from build123d import *

# Parameters (mm, degrees)
MAIN_WEB_PROFILE_W                             = 60
MAIN_WEB_PROFILE_H                             = 14
MAIN_WEB_DEPTH                                 = 4
SHOULDER_HORN_FLANGE_PROFILE_R                 = 16
SHOULDER_HORN_FLANGE_DEPTH                     = 4
ELBOW_SERVO_MOUNT_PROFILE_W                    = 48
ELBOW_SERVO_MOUNT_PROFILE_H                    = 28
ELBOW_SERVO_MOUNT_DEPTH                        = 4
SG90_BODY_CLEARANCE_START                      = -5
SG90_BODY_CLEARANCE_PROFILE_W                  = 23.8
SG90_BODY_CLEARANCE_PROFILE_H                  = 13
SG90_BODY_CLEARANCE_DEPTH                      = 97.49863387
ELBOW_TAB_FASTENERS_START                      = -50
ELBOW_TAB_FASTENERS_PROFILE_R                  = 1.3
ELBOW_TAB_FASTENERS_DEPTH                      = 142.49863387
SHOULDER_CENTER_SCREW_ACCESS_START             = -50
SHOULDER_CENTER_SCREW_ACCESS_PROFILE_R         = 4
SHOULDER_CENTER_SCREW_ACCESS_DEPTH             = 142.49863387
CABLE_TIE_HOLES_START                          = -50
CABLE_TIE_HOLES_PROFILE_R                      = 1.6
CABLE_TIE_HOLES_DEPTH                          = 142.49863387
PASSIVE_LOWER_MOUNT_BOSS_PROFILE_R             = 5
PASSIVE_LOWER_MOUNT_BOSS_DEPTH                 = 4
PASSIVE_UPPER_MOUNT_BOSS_PROFILE_R             = 5
PASSIVE_UPPER_MOUNT_BOSS_DEPTH                 = 4
PASSIVE_CHEEK_STANDOFFS_START                  = -50
PASSIVE_CHEEK_STANDOFFS_PROFILE_R              = 1.6
PASSIVE_CHEEK_STANDOFFS_DEPTH                  = 142.49863387
SHOULDER_DOWEL_SUPPORT_HUB_START               = 4
SHOULDER_DOWEL_SUPPORT_HUB_PROFILE_R           = 7
SHOULDER_DOWEL_SUPPORT_HUB_PROFILE_R_2         = 4
SHOULDER_DOWEL_SUPPORT_HUB_DEPTH               = 4
RAISED_M3_WASHER_SEATS_HEIGHT8_START           = 4
RAISED_M3_WASHER_SEATS_PCD14_PROFILE_R         = 3.5
RAISED_M3_WASHER_SEATS_HEIGHT8_DEPTH           = 4
METAL_HORN_M3_CLEARANCE_PCD14_START            = -50
METAL_HORN_M3_CLEARANCE_PCD14_PROFILE_R        = 1.6
METAL_HORN_M3_CLEARANCE_PCD14_DEPTH            = 142.760557976
RESTORE_SHOULDER_SLEEVE_BORE_START             = -50
RESTORE_SHOULDER_SLEEVE_BORE_PROFILE_R         = 4
RESTORE_SHOULDER_SLEEVE_BORE_DEPTH             = 142.760557976
FILLET1_R                                      = 7.5
LARGER_ELBOW_SERVO_MOUNT_REPLACES_SG_2_W       = 58
LARGER_ELBOW_SERVO_MOUNT_REPLACES_SG_2_H       = 30
LARGER_ELBOW_SERVO_MOUNT_REPLACES_SG90_O_DEPTH = 4
MG996R_ELBOW_BODY_CLEARANCE_START              = -5
MG996R_ELBOW_BODY_CLEARANCE_PROFILE_W          = 41.7
MG996R_ELBOW_BODY_CLEARANCE_PROFILE_H          = 20.7
MG996R_ELBOW_BODY_CLEARANCE_DEPTH              = 107.587400794
MG996R_ELBOW_TAB_FASTENERS_START               = -50
MG996R_ELBOW_TAB_FASTENERS_PROFILE_R           = 1.5
MG996R_ELBOW_TAB_FASTENERS_DEPTH               = 152.587400794
FILLET2_R                                      = 10


with BuildPart() as part:
    # Main_web_profile → Main_web (new body)
    with BuildSketch(Plane.XY):
        with Locations((30, 0)):
            Rectangle(MAIN_WEB_PROFILE_W, MAIN_WEB_PROFILE_H)
    extrude(amount=MAIN_WEB_DEPTH)

    # Shoulder_horn_flange_profile → Shoulder_horn_flange (add)
    with BuildSketch(Plane.XY):
        Circle(SHOULDER_HORN_FLANGE_PROFILE_R)
    extrude(amount=SHOULDER_HORN_FLANGE_DEPTH)

    # Elbow_servo_mount_profile → Elbow_servo_mount (add)
    with BuildSketch(Plane.XY):
        with Locations((66, 0)):
            Rectangle(ELBOW_SERVO_MOUNT_PROFILE_W, ELBOW_SERVO_MOUNT_PROFILE_H)
    extrude(amount=ELBOW_SERVO_MOUNT_DEPTH)

    # SG90_body_clearance_profile → SG90_body_clearance (cut, through all)
    with BuildSketch(Plane.XY.offset(SG90_BODY_CLEARANCE_START)):
        with Locations((65.5, 0)):
            Rectangle(SG90_BODY_CLEARANCE_PROFILE_W, SG90_BODY_CLEARANCE_PROFILE_H)
    extrude(amount=SG90_BODY_CLEARANCE_DEPTH, mode=Mode.SUBTRACT)

    # Elbow_tab_fasteners_profile → Elbow_tab_fasteners (cut, through all)
    with BuildSketch(Plane.XY.offset(ELBOW_TAB_FASTENERS_START)):
        with Locations(Location((51, 0, 0), (0, 0, 180))):
            Circle(ELBOW_TAB_FASTENERS_PROFILE_R)
        with Locations(Location((80, 0, 0), (0, 0, 180))):
            Circle(ELBOW_TAB_FASTENERS_PROFILE_R)
    extrude(amount=ELBOW_TAB_FASTENERS_DEPTH, mode=Mode.SUBTRACT)

    # Shoulder_center_screw_access_profile → Shoulder_center_screw_access (cut, through all)
    with BuildSketch(Plane.XY.offset(SHOULDER_CENTER_SCREW_ACCESS_START)):
        with Locations(Location((0, 0, 0), (0, 0, 180))):
            Circle(SHOULDER_CENTER_SCREW_ACCESS_PROFILE_R)
    extrude(amount=SHOULDER_CENTER_SCREW_ACCESS_DEPTH, mode=Mode.SUBTRACT)

    # Cable_tie_holes_profile → Cable_tie_holes (cut, through all)
    with BuildSketch(Plane.XY.offset(CABLE_TIE_HOLES_START)):
        with Locations(Location((27, -3, 0), (0, 0, 180))):
            Circle(CABLE_TIE_HOLES_PROFILE_R)
        with Locations(Location((27, 3, 0), (0, 0, 180))):
            Circle(CABLE_TIE_HOLES_PROFILE_R)
    extrude(amount=CABLE_TIE_HOLES_DEPTH, mode=Mode.SUBTRACT)

    # Passive_lower_mount_boss_profile → Passive_lower_mount_boss (add)
    with BuildSketch(Plane.XY):
        with Locations((35, -9)):
            Circle(PASSIVE_LOWER_MOUNT_BOSS_PROFILE_R)
    extrude(amount=PASSIVE_LOWER_MOUNT_BOSS_DEPTH)

    # Passive_upper_mount_boss_profile → Passive_upper_mount_boss (add)
    with BuildSketch(Plane.XY):
        with Locations((35, 9)):
            Circle(PASSIVE_UPPER_MOUNT_BOSS_PROFILE_R)
    extrude(amount=PASSIVE_UPPER_MOUNT_BOSS_DEPTH)

    # Passive_cheek_standoffs_profile → Passive_cheek_standoffs (cut, through all)
    with BuildSketch(Plane.XY.offset(PASSIVE_CHEEK_STANDOFFS_START)):
        with Locations(Location((35, -9, 0), (0, 0, 180))):
            Circle(PASSIVE_CHEEK_STANDOFFS_PROFILE_R)
        with Locations(Location((35, 9, 0), (0, 0, 180))):
            Circle(PASSIVE_CHEEK_STANDOFFS_PROFILE_R)
    extrude(amount=PASSIVE_CHEEK_STANDOFFS_DEPTH, mode=Mode.SUBTRACT)

    # Shoulder_dowel_support_hub_profile → Shoulder_dowel_support_hub (add)
    with BuildSketch(Plane.XY.offset(SHOULDER_DOWEL_SUPPORT_HUB_START)):
        Circle(SHOULDER_DOWEL_SUPPORT_HUB_PROFILE_R)
        with Locations(Location((0, 0, 0), (0, 0, 180))):
            Circle(SHOULDER_DOWEL_SUPPORT_HUB_PROFILE_R_2, mode=Mode.SUBTRACT)
    extrude(amount=SHOULDER_DOWEL_SUPPORT_HUB_DEPTH)

    # Raised_M3_washer_seats_PCD14_profile → Raised_M3_washer_seats_height8 (add)
    with BuildSketch(Plane.XY.offset(RAISED_M3_WASHER_SEATS_HEIGHT8_START)):
        with Locations((7, 0)):
            Circle(RAISED_M3_WASHER_SEATS_PCD14_PROFILE_R)
        with Locations((-7, 0)):
            Circle(RAISED_M3_WASHER_SEATS_PCD14_PROFILE_R)
        with Locations((0, 7)):
            Circle(RAISED_M3_WASHER_SEATS_PCD14_PROFILE_R)
        with Locations((0, -7)):
            Circle(RAISED_M3_WASHER_SEATS_PCD14_PROFILE_R)
    extrude(amount=RAISED_M3_WASHER_SEATS_HEIGHT8_DEPTH)

    # Metal_horn_M3_clearance_PCD14_profile → Metal_horn_M3_clearance_PCD14 (cut, through all)
    with BuildSketch(Plane.XY.offset(METAL_HORN_M3_CLEARANCE_PCD14_START)):
        with Locations(Location((7, 0, 0), (0, 0, 180))):
            Circle(METAL_HORN_M3_CLEARANCE_PCD14_PROFILE_R)
        with Locations(Location((-7, 0, 0), (0, 0, 180))):
            Circle(METAL_HORN_M3_CLEARANCE_PCD14_PROFILE_R)
        with Locations(Location((0, 7, 0), (0, 0, 180))):
            Circle(METAL_HORN_M3_CLEARANCE_PCD14_PROFILE_R)
        with Locations(Location((0, -7, 0), (0, 0, 180))):
            Circle(METAL_HORN_M3_CLEARANCE_PCD14_PROFILE_R)
    extrude(amount=METAL_HORN_M3_CLEARANCE_PCD14_DEPTH, mode=Mode.SUBTRACT)

    # Restore_shoulder_sleeve_bore_profile → Restore_shoulder_sleeve_bore (cut, through all)
    with BuildSketch(Plane.XY.offset(RESTORE_SHOULDER_SLEEVE_BORE_START)):
        with Locations(Location((0, 0, 0), (0, 0, 180))):
            Circle(RESTORE_SHOULDER_SLEEVE_BORE_PROFILE_R)
    extrude(amount=RESTORE_SHOULDER_SLEEVE_BORE_DEPTH, mode=Mode.SUBTRACT)

    # Fillet1
    # the kernel refuses this fillet: 7.5 mm, written as the material it takes off along each edge
    with BuildSketch(Plane(origin=(42, -14, -18.708286934), x_dir=(0, 1, 0), z_dir=(0, 0, 1))) as fillet1_piece_1:
        with BuildLine():
            CenterArc((7.5, -7.483314774), FILLET1_R, 93.822553729, 86.177446271)
            Line((0, -7.483314774), (-0.15, -7.483314774))
            Line((-0.15, -7.483314774), (-0.15, 0))
            Line((-0.15, 0), (0, 0.15))
            ThreePointArc((0, 0.15), (3.5, 0.15), (6.99, 0.149666295))
            Line((6.99, 0.149666295), (7, 0))
        make_face()
    extrude(amount=41.416573868, mode=Mode.SUBTRACT)
    with BuildSketch(Plane(origin=(90, -14, -18.75), x_dir=(-1, 0, 0), z_dir=(0, 0, 1)), Plane(origin=(90, 14, -18.75), x_dir=(0, -1, 0), z_dir=(0, 0, 1))) as fillet1_piece_2:
        with BuildLine():
            CenterArc((FILLET1_R, -FILLET1_R), FILLET1_R, 90, 90)
            Line((0, -FILLET1_R), (-FILLET1_R * 0.02, -FILLET1_R))
            Line((-FILLET1_R * 0.02, -FILLET1_R), (-FILLET1_R * 0.02, FILLET1_R * 0.02))
            Line((-FILLET1_R * 0.02, FILLET1_R * 0.02), (FILLET1_R, FILLET1_R * 0.02))
            Line((FILLET1_R, FILLET1_R * 0.02), (FILLET1_R, 0))
        make_face()
    extrude(amount=41.5, mode=Mode.SUBTRACT)
    with BuildSketch(Plane(origin=(42, 14, -18.708286934), x_dir=(0, -1, 0), z_dir=(0, 0, 1))) as fillet1_piece_3:
        with BuildLine():
            CenterArc((7.5, 7.483314774), FILLET1_R, 180, 86.177446271)
            Line((0, 7.483314774), (-0.15, 7.483314774))
            Line((-0.15, 7.483314774), (-0.15, 0))
            Line((-0.15, 0), (0, -0.15))
            ThreePointArc((0, -0.15), (3.5, -0.15), (6.99, -0.149666295))
            Line((6.99, -0.149666295), (7, 0))
        make_face()
    extrude(amount=41.416573868, mode=Mode.SUBTRACT)

    # Larger_elbow_servo_mount_replaces_SG 2 → Larger_elbow_servo_mount_replaces_SG90_o (add)
    with BuildSketch(Plane.XY):
        with Locations((71, 0)):
            Rectangle(LARGER_ELBOW_SERVO_MOUNT_REPLACES_SG_2_W, LARGER_ELBOW_SERVO_MOUNT_REPLACES_SG_2_H)
    extrude(amount=LARGER_ELBOW_SERVO_MOUNT_REPLACES_SG90_O_DEPTH)

    # MG996R_elbow_body_clearance_profile → MG996R_elbow_body_clearance (cut, through all)
    with BuildSketch(Plane.XY.offset(MG996R_ELBOW_BODY_CLEARANCE_START)):
        with Locations((70.35, 0)):
            Rectangle(MG996R_ELBOW_BODY_CLEARANCE_PROFILE_W, MG996R_ELBOW_BODY_CLEARANCE_PROFILE_H)
    extrude(amount=MG996R_ELBOW_BODY_CLEARANCE_DEPTH, mode=Mode.SUBTRACT)

    # MG996R_elbow_tab_fasteners_profile → MG996R_elbow_tab_fasteners (cut, through all)
    with BuildSketch(Plane.XY.offset(MG996R_ELBOW_TAB_FASTENERS_START)):
        with Locations(Location((47, -5, 0), (0, 0, 180))):
            Circle(MG996R_ELBOW_TAB_FASTENERS_PROFILE_R)
        with Locations(Location((47, 5, 0), (0, 0, 180))):
            Circle(MG996R_ELBOW_TAB_FASTENERS_PROFILE_R)
        with Locations(Location((94, -5, 0), (0, 0, 180))):
            Circle(MG996R_ELBOW_TAB_FASTENERS_PROFILE_R)
        with Locations(Location((94, 5, 0), (0, 0, 180))):
            Circle(MG996R_ELBOW_TAB_FASTENERS_PROFILE_R)
    extrude(amount=MG996R_ELBOW_TAB_FASTENERS_DEPTH, mode=Mode.SUBTRACT)

    # Fillet2
    # the kernel refuses this fillet: 10 mm, written as the material it takes off along each edge
    with BuildSketch(Plane(origin=(42, 15, -24.494897428), x_dir=(1, 0, 0), z_dir=(0, 0, 1))) as fillet2_piece_1:
        with BuildLine():
            CenterArc((9.797958971, -10), FILLET2_R, 90, 78.463040967)
            Line((0, -8), (-0.195959179, -7.96))
            ThreePointArc((-0.195959179, -7.96), (-0.2, -4), (-0.2, 0))
            Line((-0.2, 0), (0, 0.2))
            Line((0, 0.2), (9.797958971, 0.2))
            Line((9.797958971, 0.2), (9.797958971, 0))
        make_face()
    extrude(amount=52.989794856, mode=Mode.SUBTRACT)
    with BuildSketch(Plane(origin=(42, -15, -24.494897428), x_dir=(0, 1, 0), z_dir=(0, 0, 1))) as fillet2_piece_2:
        with BuildLine():
            CenterArc((10, -9.797958971), FILLET2_R, 101.536959033, 78.463040967)
            Line((0, -9.797958971), (-0.2, -9.797958971))
            Line((-0.2, -9.797958971), (-0.2, 0))
            Line((-0.2, 0), (0, 0.2))
            ThreePointArc((0, 0.2), (4, 0.2), (7.96, 0.195959179))
            Line((7.96, 0.195959179), (8, 0))
        make_face()
    extrude(amount=52.989794856, mode=Mode.SUBTRACT)
    with BuildSketch(Plane(origin=(100, -15, -25), x_dir=(-1, 0, 0), z_dir=(0, 0, 1)), Plane(origin=(100, 15, -25), x_dir=(0, -1, 0), z_dir=(0, 0, 1))) as fillet2_piece_3:
        with BuildLine():
            CenterArc((FILLET2_R, -FILLET2_R), FILLET2_R, 90, 90)
            Line((0, -FILLET2_R), (-FILLET2_R * 0.02, -FILLET2_R))
            Line((-FILLET2_R * 0.02, -FILLET2_R), (-FILLET2_R * 0.02, FILLET2_R * 0.02))
            Line((-FILLET2_R * 0.02, FILLET2_R * 0.02), (FILLET2_R, FILLET2_R * 0.02))
            Line((FILLET2_R, FILLET2_R * 0.02), (FILLET2_R, 0))
        make_face()
    extrude(amount=54, mode=Mode.SUBTRACT)


solid = part.part
For this review, take the finished solid that the model builds, in its own axes (mm). A direction names the side the tool comes from. Round coordinates to 2 decimals unless told otherwise and drop trailing zeros. Write each loop counter-clockwise with the first axis right and the second up, starting at its lowest first coordinate (ties: lowest second). Pieces come first, ordered by that corner, then holes. Notation, with made-up numbers: (-21, 44) -> (8, 44) arc R20 cw to (8, 73) -> close; hole circle Ø8 at (42.5, 37). An arc over 180 degrees is marked (long way). Use CSV: the item, a comma, the result in double quotes.
(1) For faces 5 (the face through (97.15, 11.99, 1.97)), 6 (the face through (10.5, -0.1, 6)), 7 (the face through (70, -10.35, 2)), list the 3-axis set-ups (+Z, -Z, +X, -X, +Y, -Y) from which the entire face can be reached by the end or side of a thin tool; tool diameter is ignored.
Computed values:
face 5,"+Z, -Z, +X, +Y"
face 6,"+Z"
face 7,"+Z, -Z"
(2) Clearance check with flat-ended pins moving along their axes: P1, Ø1.5, axis at x = 68.5, z = 1, coming from the -Y side; P2, Ø16, axis at x = 38, y = -0.5, coming from the +Z side; P3, Ø1.2, axis at x = 75.5, z = 1.5, coming from the +Y side. State where each tip first meets the part, or that it passes through.
Computed values:
P1,"y = -15"
P2,"z = 4"
P3,"y = 15"
(3) To check wall thickness, follow L1, parallel to Y at x = 79.5, z = 3; L2, parallel to Y at x = 35, z = 2.2; L3, parallel to X at y = -1, z = 7.5. State the ranges of each line that lie inside material, in increasing order. Write a range as [from, to].
Computed values:
L1,"[-15, -10.35], [10.35, 15]"
L2,"[-14, -10.6], [-7.4, 7.4], [10.6, 14]"
L3,"[-10.35, -8.25], [-5.75, -3.87], [3.87, 5.75], [8.25, 10.35]"
(4) Consider section A-A, the plane x = 86.5. Give the boundary of the cut face in (y, z), plus the area to 3 significant figures.
Computed values:
outline,"(-15, 0) -> (-10.35, 0) -> (-10.35, 4) -> (-15, 4) -> close; (10.35, 0) -> (15, 0) -> (15, 4) -> (10.35, 4) -> close"
area,"37.2 mm²"
(5) Consider section D-D, the plane z = 7. Give the boundary of the cut face in (x, y) (3 decimals), plus the area to 3 significant figures.
Computed values:
outline,"(-6.125, -3.389) arc R7 ccw to (-3.389, -6.125) arc R3.5 ccw (long way) to (3.389, -6.125) arc R7 ccw to (6.125, -3.389) arc R3.5 ccw (long way) to (6.125, 3.389) arc R7 ccw to (3.389, 6.125) arc R3.5 ccw (long way) to (-3.389, 6.125) arc R7 ccw to (-6.125, 3.389) arc R3.5 ccw (long way) to start; hole circle Ø3.2 at (-7, 0); hole circle Ø8 at (0, 0); hole circle Ø3.2 at (0, -7); hole circle Ø3.2 at (0, 7); hole circle Ø3.2 at (7, 0)"
area,"157 mm²"
(6) Draft analysis for pull direction Y (two halves, no side actions). For faces 1 (the face through (-5.4, -0.07, 3.94)), 2 (the face through (0.867, 3.905, 3.944)), 3 (the face through (41, 0, 4)), 4 (the face through (-10.5, 0.1, 6)), state which applies: +Y half, -Y half, draft (parallel to the pull), parting line (faces both ways), or undercut.
Computed values:
face 1,"undercut"
face 2,"undercut"
face 3,"draft"
face 4,"parting line"
(7) Consider section C-C, the plane x = 0.5. Give the boundary of the cut face in (y, z).
Computed values:
outline,"(-15.99, 0) -> (-8.52, 0) -> (-8.52, 8) -> (-10.46, 8) -> (-10.46, 4) -> (-15.99, 4) -> close; (-5.48, 0) -> (-3.97, 0) -> (-3.97, 8) -> (-5.48, 8) -> close; (3.97, 0) -> (5.48, 0) -> (5.48, 8) -> (3.97, 8) -> close; (8.52, 0) -> (15.99, 0) -> (15.99, 4) -> (10.46, 4) -> (10.46, 8) -> (8.52, 8) -> close"
(8) Consider section B-B, the plane z = 1.5. Give the number of separate pieces and of enclosed holes in the cut face, plus the area to 3 significant figures.
Computed values:
separate pieces,"1"
enclosed holes,"14"
area,"1,940 mm²"
